Design review of the part built by this model. Coordinates are the model's own, in mm. A direction names the side the tool comes from. Coordinates: 2 decimals unless noted, no trailing zeros. Order: outer loops, then holes, each group sorted by start corner. A loop starts at its lowest first (then second) coordinate and runs counter-clockwise, first axis right, second up. Notation, with made-up numbers: (61, 11) -> (90, 11) arc R6 ccw to (90, 16) -> close; hole circle Ø11 at (-8, 77). An arc over 180 degrees is marked (long way). Write item = value, one per line.
```python
from build123d import *

# Parameters (mm, degrees)
SKETCH1_W               = 673.1
SKETCH1_H               = 237.6932
SKETCH1_R               = 38.89375
BOSS_EXTRUDE1_DEPTH     = 9.525
SKETCH2_W               = 673.1
SKETCH2_H               = 4.699
CUT_EXTRUDE1_DEPTH      = 10.16
SKETCH3_W               = 7.9375
SKETCH3_H               = 209.1182
BOSS_EXTRUDE2_DEPTH     = 19.05
FILLET1_R               = 6.35
CUT_EXTRUDE2_DEPTH      = 692.395195502
CUT_EXTRUDE2_DEPTH_BACK = 692.395195502
CUT_EXTRUDE3_START      = -19.05
CUT_EXTRUDE3_DEPTH      = 7.9375
CUT_EXTRUDE4_DEPTH      = 365.9096525
CUT_EXTRUDE4_DEPTH_BACK = 365.9096525
SKETCH6_R               = 9.525
SKETCH6_R_2             = 38
SKETCH6_R_3             = 2.159
CUT_EXTRUDE5_DEPTH      = 365.536524388
CUT_EXTRUDE5_DEPTH_BACK = 365.536524388
SKETCH8_W               = 7
SKETCH8_H               = 7.9375


with BuildPart() as part:
    # Sketch1 → Boss-Extrude1 (new, symmetric)
    with BuildSketch(Plane(origin=(0, 0, 0), x_dir=(1, 0, 0), z_dir=(0, 1, 0))):
        Rectangle(SKETCH1_W, SKETCH1_H)
        with Locations(Location((-254, -53.8734, 0), (0, 0, 90))):
            Circle(SKETCH1_R, mode=Mode.SUBTRACT)
        with Locations(Location((254, -53.8734, 0), (0, 0, 90))):
            Circle(SKETCH1_R, mode=Mode.SUBTRACT)
    extrude(amount=BOSS_EXTRUDE1_DEPTH, both=True)

    # Sketch2 → Cut-Extrude1 (cut)
    with BuildSketch(Plane(origin=(0, 9.525, 0), x_dir=(1, 0, 0), z_dir=(0, 1, 0))):
        with Locations((0, -110.2395052)):
            Rectangle(SKETCH2_W, SKETCH2_H)
    extrude(amount=-CUT_EXTRUDE1_DEPTH, mode=Mode.SUBTRACT)

    # Sketch3 → Boss-Extrude2 (add)
    with BuildSketch(Plane(origin=(0, 9.525, 0), x_dir=(1, 0, 0), z_dir=(0, 1, 0))):
        with Locations((-340.51875, 0)):
            Rectangle(SKETCH3_W, SKETCH3_H)
        with Locations((340.51875, 0)):
            Rectangle(SKETCH3_W, SKETCH3_H)
    extrude(amount=-BOSS_EXTRUDE2_DEPTH)

    # Fillet1
    # the kernel refuses this fillet: 6.35 mm, written as the material it adds along each edge
    with BuildSketch(Plane(origin=(336.55, 9.525, -104.5591), x_dir=(0, 0, -1), z_dir=(0, -1, 0))) as fillet1_piece_1:
        with BuildLine():
            CenterArc((FILLET1_R, FILLET1_R), FILLET1_R, 180, 90)
            Line((0, FILLET1_R), (0, 0))
            Line((0, 0), (FILLET1_R, 0))
        make_face()
    extrude(amount=19.05)
    with BuildSketch(Plane(origin=(336.55, 9.525, 104.5591), x_dir=(0, 0, 1), z_dir=(0, -1, 0))) as fillet1_piece_2_section:
        with BuildLine():
            CenterArc((FILLET1_R, -FILLET1_R), FILLET1_R, 90, 90)
            Line((0, -FILLET1_R), (0, 0))
            Line((0, 0), (FILLET1_R, 0))
        make_face()
    fillet1_piece_2 = extrude(amount=19.05, mode=Mode.PRIVATE)
    fillet1_piece_2 = split(fillet1_piece_2, bisect_by=Plane(origin=(338.149651187, -0.635, 105.638113303), z_dir=(0, 1, 0)), keep=Keep.TOP, mode=Mode.PRIVATE)
    fillet1_piece_2 = split(fillet1_piece_2, bisect_by=Plane(origin=(338.149651187, 4.445, 107.8900052), z_dir=(0, 0, -1)), keep=Keep.TOP, mode=Mode.PRIVATE)
    add(fillet1_piece_2)
    with BuildSketch(Plane(origin=(336.55, 9.525, 104.5591), x_dir=(0, 0, 1), z_dir=(0, -1, 0))) as fillet1_piece_3_section:
        with BuildLine():
            CenterArc((FILLET1_R, -FILLET1_R), FILLET1_R, 90, 90)
            Line((0, -FILLET1_R), (0, 0))
            Line((0, 0), (FILLET1_R, 0))
        make_face()
    fillet1_piece_3 = extrude(amount=19.05, mode=Mode.PRIVATE)
    fillet1_piece_3 = split(fillet1_piece_3, bisect_by=Plane(origin=(336.678320254, -0.635, 108.894134697), z_dir=(0, -1, 0)), keep=Keep.TOP, mode=Mode.PRIVATE)
    fillet1_piece_3 = split(fillet1_piece_3, bisect_by=Plane(origin=(336.678320254, -5.08, 107.8900052), z_dir=(0, 0, 1)), keep=Keep.TOP, mode=Mode.PRIVATE)
    add(fillet1_piece_3)
    with BuildSketch(Plane(origin=(336.55, 9.525, 104.5591), x_dir=(0, 0, 1), z_dir=(0, -1, 0))) as fillet1_piece_4_section:
        with BuildLine():
            CenterArc((FILLET1_R, -FILLET1_R), FILLET1_R, 90, 90)
            Line((0, -FILLET1_R), (0, 0))
            Line((0, 0), (FILLET1_R, 0))
        make_face()
    fillet1_piece_4 = extrude(amount=19.05, mode=Mode.PRIVATE)
    fillet1_piece_4 = split(fillet1_piece_4, bisect_by=Plane(origin=(338.149651187, -0.635, 105.638113303), z_dir=(0, -1, 0)), keep=Keep.TOP, mode=Mode.PRIVATE)
    fillet1_piece_4 = split(fillet1_piece_4, bisect_by=Plane(origin=(338.149651187, -5.08, 107.8900052), z_dir=(0, 0, -1)), keep=Keep.TOP, mode=Mode.PRIVATE)
    add(fillet1_piece_4)
    with BuildSketch(Plane(origin=(-336.55, 9.525, -104.5591), x_dir=(0, 0, -1), z_dir=(0, -1, 0))) as fillet1_piece_5:
        with BuildLine():
            CenterArc((FILLET1_R, -FILLET1_R), FILLET1_R, 90, 90)
            Line((0, -FILLET1_R), (0, 0))
            Line((0, 0), (FILLET1_R, 0))
        make_face()
    extrude(amount=19.05)
    with BuildSketch(Plane(origin=(-336.55, 9.525, 104.5591), x_dir=(0, 0, 1), z_dir=(0, -1, 0))) as fillet1_piece_6_section:
        with BuildLine():
            CenterArc((FILLET1_R, FILLET1_R), FILLET1_R, 180, 90)
            Line((0, FILLET1_R), (0, 0))
            Line((0, 0), (FILLET1_R, 0))
        make_face()
    fillet1_piece_6 = extrude(amount=19.05, mode=Mode.PRIVATE)
    fillet1_piece_6 = split(fillet1_piece_6, bisect_by=Plane(origin=(-338.149651187, 4.445, 107.8900052), z_dir=(0, 0, -1)), keep=Keep.TOP, mode=Mode.PRIVATE)
    fillet1_piece_6 = split(fillet1_piece_6, bisect_by=Plane(origin=(-338.149651187, -0.635, 105.638113303), z_dir=(0, 1, 0)), keep=Keep.TOP, mode=Mode.PRIVATE)
    add(fillet1_piece_6)
    with BuildSketch(Plane(origin=(-336.55, 9.525, 104.5591), x_dir=(0, 0, 1), z_dir=(0, -1, 0))) as fillet1_piece_7_section:
        with BuildLine():
            CenterArc((FILLET1_R, FILLET1_R), FILLET1_R, 180, 90)
            Line((0, FILLET1_R), (0, 0))
            Line((0, 0), (FILLET1_R, 0))
        make_face()
    fillet1_piece_7 = extrude(amount=19.05, mode=Mode.PRIVATE)
    fillet1_piece_7 = split(fillet1_piece_7, bisect_by=Plane(origin=(-336.678320254, -5.08, 107.8900052), z_dir=(0, 0, 1)), keep=Keep.TOP, mode=Mode.PRIVATE)
    fillet1_piece_7 = split(fillet1_piece_7, bisect_by=Plane(origin=(-336.678320254, -0.635, 108.894134697), z_dir=(0, -1, 0)), keep=Keep.TOP, mode=Mode.PRIVATE)
    add(fillet1_piece_7)
    with BuildSketch(Plane(origin=(-336.55, 9.525, 104.5591), x_dir=(0, 0, 1), z_dir=(0, -1, 0))) as fillet1_piece_8_section:
        with BuildLine():
            CenterArc((FILLET1_R, FILLET1_R), FILLET1_R, 180, 90)
            Line((0, FILLET1_R), (0, 0))
            Line((0, 0), (FILLET1_R, 0))
        make_face()
    fillet1_piece_8 = extrude(amount=19.05, mode=Mode.PRIVATE)
    fillet1_piece_8 = split(fillet1_piece_8, bisect_by=Plane(origin=(-338.149651187, -5.08, 107.8900052), z_dir=(0, 0, -1)), keep=Keep.TOP, mode=Mode.PRIVATE)
    fillet1_piece_8 = split(fillet1_piece_8, bisect_by=Plane(origin=(-338.149651187, -0.635, 105.638113303), z_dir=(0, -1, 0)), keep=Keep.TOP, mode=Mode.PRIVATE)
    add(fillet1_piece_8)

    # Sketch4 → Cut-Extrude2 (cut, two sides: drawn at the far end of the back side and taken through both)
    with BuildSketch(Plane(origin=(336.55, 0, 0), x_dir=(0, 0, -1), z_dir=(1, 0, 0)).offset(-CUT_EXTRUDE2_DEPTH_BACK)):
        Polygon((118.8466, -9.525), (115.487571018, 9.525), (118.8466, 9.525), align=None)
    extrude(amount=CUT_EXTRUDE2_DEPTH + CUT_EXTRUDE2_DEPTH_BACK, mode=Mode.SUBTRACT)

    # Sketch5 → Cut-Extrude3 (cut)
    with BuildSketch(Plane.XZ.offset(9.525).offset(CUT_EXTRUDE3_START)):
        with BuildLine():
            Line((-323.05625, -9.201160668), (323.05625, -9.201160668))
            ThreePointArc((323.05625, -9.201160668), (331.05725, -17.202160668), (323.05625, -25.203160668))
            Line((323.05625, -25.203160668), (-323.05625, -25.203160668))
            ThreePointArc((-323.05625, -25.203160668), (-331.05725, -17.202160668), (-323.05625, -9.201160668))
        make_face()
    extrude(amount=CUT_EXTRUDE3_DEPTH, mode=Mode.SUBTRACT)

    # Sketch6 → Cut-Extrude4 (cut, two sides: drawn at the far end of the back side and taken through both)
    with BuildSketch(Plane(origin=(0, 9.525, 0), x_dir=(1, 0, 0), z_dir=(0, 1, 0)).offset(-CUT_EXTRUDE4_DEPTH_BACK)):
        with Locations(Location((-319.0875, 68.0466, 0), (0, 0, 270))):
            Circle(SKETCH6_R)
        with Locations(Location((319.0875, 68.0466, 0), (0, 0, 270))):
            Circle(SKETCH6_R)
        with Locations(Location((127, 71.2216, 0), (0, 0, 270))):
            Circle(SKETCH6_R_2)
        with Locations(Location((-127, 71.2216, 0), (0, 0, 270))):
            Circle(SKETCH6_R_2)
        with Locations(Location((162.75, 106.9716, 0), (0, 0, 270))):
            Circle(SKETCH6_R_3)
        with Locations(Location((162.75, 35.4716, 0), (0, 0, 270))):
            Circle(SKETCH6_R_3)
        with Locations(Location((91.25, 35.4716, 0), (0, 0, 270))):
            Circle(SKETCH6_R_3)
        with Locations(Location((91.25, 106.9716, 0), (0, 0, 270))):
            Circle(SKETCH6_R_3)
        with Locations(Location((-91.25, 106.9716, 0), (0, 0, 90))):
            Circle(SKETCH6_R_3)
        with Locations(Location((-91.25, 35.4716, 0), (0, 0, 90))):
            Circle(SKETCH6_R_3)
        with Locations(Location((-162.75, 35.4716, 0), (0, 0, 90))):
            Circle(SKETCH6_R_3)
        with Locations(Location((-162.75, 106.9716, 0), (0, 0, 90))):
            Circle(SKETCH6_R_3)
    extrude(amount=CUT_EXTRUDE4_DEPTH + CUT_EXTRUDE4_DEPTH_BACK, mode=Mode.SUBTRACT)

    # Sketch8 → Cut-Extrude5 (cut, two sides: drawn at the far end of the back side and taken through both)
    with BuildSketch(Plane(origin=(0, 0, 0), x_dir=(0, 0, -1), z_dir=(1, 0, 0)).offset(-CUT_EXTRUDE5_DEPTH_BACK)):
        with Locations((4.6533886, -5.55625)):
            Rectangle(SKETCH8_W, SKETCH8_H)
    extrude(amount=CUT_EXTRUDE5_DEPTH + CUT_EXTRUDE5_DEPTH_BACK, mode=Mode.SUBTRACT)


solid = part.part
```
(1) For faces 1 (the flat face through (5, 1.588, -17)), 2 (the flat face through (-5, -9.525, 60)), list the 3-axis set-ups (+Z, -Z, +X, -X, +Y, -Y) from which the entire face can be reached by the end or side of a thin tool; tool diameter is ignored.
Report:
face_1 = +Y
face_2 = +Z, -Z, +X, -X, -Y
(2) We need section A-A (x = 127). Write out the cut boundary in (y, z) (1 decimal), and give its area (3 significant figures).
Report:
outline = (-9.5, -118.8) -> (9.5, -115.5) -> (9.5, -109.2) -> (-9.5, -109.2) -> close; (-9.5, -33.2) -> (9.5, -33.2) -> (9.5, -25.2) -> (1.6, -25.2) -> (1.6, -9.2) -> (9.5, -9.2) -> (9.5, 107.9) -> (-0.6, 107.9) -> (-0.6, 112.6) -> (9.5, 112.6) -> (9.5, 118.8) -> (-9.5, 118.8) -> (-9.5, -1.2) -> (-1.6, -1.2) -> (-1.6, -8.2) -> (-9.5, -8.2) -> close
area = 2,820 mm²
(3) We need section C-C (x = -301). Write out the cut boundary in (y, z) (1 decimal).
Report:
outline = (-9.5, -118.8) -> (9.5, -115.5) -> (9.5, -25.2) -> (1.6, -25.2) -> (1.6, -9.2) -> (9.5, -9.2) -> (9.5, 107.9) -> (-0.6, 107.9) -> (-0.6, 112.6) -> (9.5, 112.6) -> (9.5, 118.8) -> (-9.5, 118.8) -> (-9.5, -1.2) -> (-1.6, -1.2) -> (-1.6, -8.2) -> (-9.5, -8.2) -> close
(4) The part is to be moulded in two halves that separate along X. For faces 3 (the cylindrical face through (-309.644, -0.133, -69.287)), 4 (the cylindrical face through (291.97, -0.13, 62.3)), 5 (the flat face through (-344.488, 0, 1)), 6 (the flat face through (-5, -9.525, -63)), say which applies: released by +X, released by -X, zero draft, split by the parting line, or undercut.
Report:
face_3 = undercut
face_4 = undercut
face_5 = released by -X
face_6 = zero draft
(5) For L1, parallel to Z at x = 127, y = 3.75; L2, parallel to Z at x = 283.5, y = -2.25; L3, parallel to X at y = -7, z = 79, list the stretches that pass through material, from the lowest coordinate up.
Report:
L1 = -116.51 to -109.22, -33.22 to -25.2, -9.2 to 107.89, 112.59 to 118.85
L2 = -117.56 to -8.15, -1.15 to 28.53, 79.22 to 118.85
L3 = -344.49 to -283.69, -224.31 to 224.31, 283.69 to 344.49
(6) We need section D-D (x = -149.5). Write out the cut boundary in (y, z) (1 decimal).
Report:
outline = (-9.5, -118.8) -> (9.5, -115.5) -> (9.5, -101.8) -> (-9.5, -101.8) -> close; (-9.5, -40.6) -> (9.5, -40.6) -> (9.5, -25.2) -> (1.6, -25.2) -> (1.6, -9.2) -> (9.5, -9.2) -> (9.5, 107.9) -> (-0.6, 107.9) -> (-0.6, 112.6) -> (9.5, 112.6) -> (9.5, 118.8) -> (-9.5, 118.8) -> (-9.5, -1.2) -> (-1.6, -1.2) -> (-1.6, -8.2) -> (-9.5, -8.2) -> close
(7) We need section B-B (y = 6.5). Give the number of separate pieces and of enclosed holes in the cut face, and give its area (3 significant figures).
Report:
separate_pieces = 2
enclosed_holes = 15
area = 128,000 mm²
(8) Insertion check: pin 1 (0.8 mm diameter, centred on x = 343.5, y = 4.5, fed in from -Z); pin 2 (1.7 mm diameter, centred on x = 344, y = 4, fed in from +Z); pin 3 (8.5 mm diameter, centred on y = -4.5, z = -116, fed in from -X). Each pin has a flat end and moves straight along its axis. Give the tip position at first contact, or say it passes through.
Report:
pin_1 = -104.56
pin_2 = 104.56
pin_3 = -336.55
